Could you check a few things on this model? Use its own coordinates, in mm. Face numbers are marked on the shaded views. Coordinates: 2 decimals unless noted, no trailing zeros. Order: outer loops, then holes, each group sorted by start corner. A loop starts at its lowest first (then second) coordinate and runs counter-clockwise, first axis right, second up. Notation, with made-up numbers: (89, 50) - (145, 50) arc R15 ccw to (145, 66) - close; hole circle Ø5 at (10.5, 42). An arc over 180 degrees is marked (long way). One line per item, written item: value.
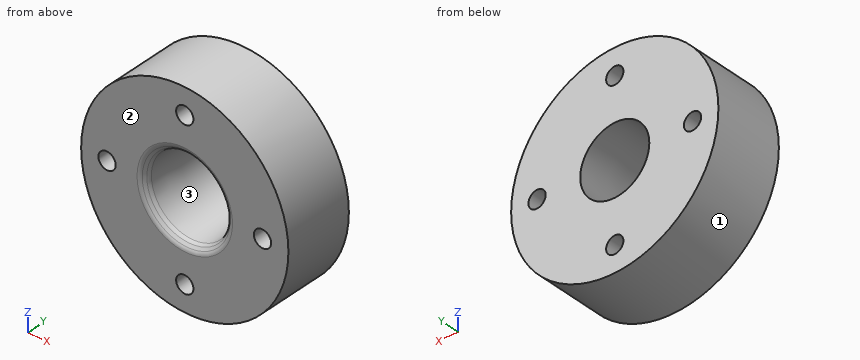
from build123d import *

# Parameters (mm, degrees)
FILLET1_R          = 2
SKETCH3_R          = 3.175
CUT_EXTRUDE1_DEPTH = 74.231772476


with BuildPart() as part:
    # Sketch2 → Revolve2 (revolve)
    with BuildSketch(Plane.XY, mode=Mode.PRIVATE) as revolve2_sk:
        Polygon((19.05, -12.7), (-2.29475363, -12.7), (-2.320408163, -12.7), (-4.320233699, -10.701915819), (-6.35, 12.7), (19.05, 12.7), align=None)
    revolve(revolve2_sk.sketch.rotate(Axis((-19.05, 12.7, 0), (0, -1, 0)), 180), axis=Axis((-19.05, 12.7, 0), (0, -1, 0)))

    # Fillet1
    fillet1_edges = [part.edges().sort_by_distance(p)[0] for p in [
        (-4.320233699, -10.701915819, 0),
        (-2.320408163, -12.7, 0),
    ]]
    fillet(fillet1_edges, radius=FILLET1_R)

    # Sketch3 → Cut-Extrude1 (cut, through all)
    with BuildSketch(Plane(origin=(0, 12.7, 0), x_dir=(1, 0, 0), z_dir=(0, 1, 0))):
        with Locations(Location((-19.05, 28.575, 0), (0, 0, 180))):
            Circle(SKETCH3_R)
        with Locations(Location((9.525, 0, 0), (0, 0, 180))):
            Circle(SKETCH3_R)
        with Locations(Location((-19.05, -28.575, 0), (0, 0, 180))):
            Circle(SKETCH3_R)
        with Locations(Location((-47.625, 0, 0), (0, 0, 180))):
            Circle(SKETCH3_R)
    extrude(amount=-CUT_EXTRUDE1_DEPTH, mode=Mode.SUBTRACT)


solid = part.part
Item 1: I want a section at A-A on x = -47. Please give me the cut outline in (y, z).
Conclusion:
outline: (-12.7, -25.89) - (12.7, -25.89) - (12.7, -3.11) - (-12.7, -3.11) - close; (-12.7, 3.11) - (12.7, 3.11) - (12.7, 25.89) - (-12.7, 25.89) - close
Item 2: I'm going to push flat-ended pins straight in: pin 1 Ø5 at (x, z) = (-47.625, 0) entering from -Y; pin 2 Ø3 at (x, y) = (5.5, -8) entering from +Z; pin 3 Ø12 at (y, z) = (6.5, 21.5) entering from +X; pin 4 Ø3 at (x, y) = (-30, 4.5) entering from -Z. Where does each tip first touch, or does it pass through?
Conclusion:
pin 1: through
pin 2: z = 30.34
pin 3: x = 15.75
pin 4: z = -36.91
Item 3: I want a section at B-B on z = 0. Give the number of separate pieces and of enclosed holes in the cut face, then the cut area to 3 significant figures.
Conclusion:
separate pieces: 4
enclosed holes: 0
area: 908 mm²
Item 4: If I drill on probe 1 along Z at (x, y) = (-19.05, 3.75); probe 2 along Z at (x, y) = (-29.5, -8); probe 3 along Z at (x, y) = (-48, -0.75), over which ranges is the centre line in solid material (lowest first)?
Conclusion:
probe 1: -38.1 to -31.75, -25.4 to -13.48, 13.48 to 25.4, 31.75 to 38.1
probe 2: -36.64 to -10.05, 10.05 to 36.64
probe 3: -24.77 to -3.15, 3.15 to 24.77
Item 5: Thinking about a two-plate mould opening in Z: for the marked faces 1, 2 and 3, which applies, pulls with the +Z half, pulls with the -Z half, needs draft (parallel to the pull), parting line crosses it, or undercut?
Conclusion:
face 1: parting line crosses it
face 2: needs draft
face 3: undercut
Item 6: I want a section at C-C on y = 3. Please give me the cut outline in (x, z) (3 decimals).
Conclusion:
outline: circle Ø76.2 at (-19.05, 0); hole circle Ø6.35 at (-47.625, 0); hole circle Ø27.083 at (-19.05, 0); hole circle Ø6.35 at (-19.05, -28.575); hole circle Ø6.35 at (-19.05, 28.575); hole circle Ø6.35 at (9.525, 0)
